Source: three-view drawing plus pictorial views. Frame: mm from the lowest corner of the part. A direction names the side the tool comes from. Give positions to 0.01 mm unless a question says otherwise; leave off trailing zeros. Loops run counter-clockwise (first coordinate to the right, second up) from the corner with the lowest first, then second, coordinate; pieces in that order, holes last. Notation, with made-up numbers: (-17, 82) -> (-10, 82) arc R23 cw to (-10, 101) -> close; hole circle Ø6 at (44.25, -11.5). An arc over 180 degrees is marked (long way). One line per item, written item: value. Start each with the question number.
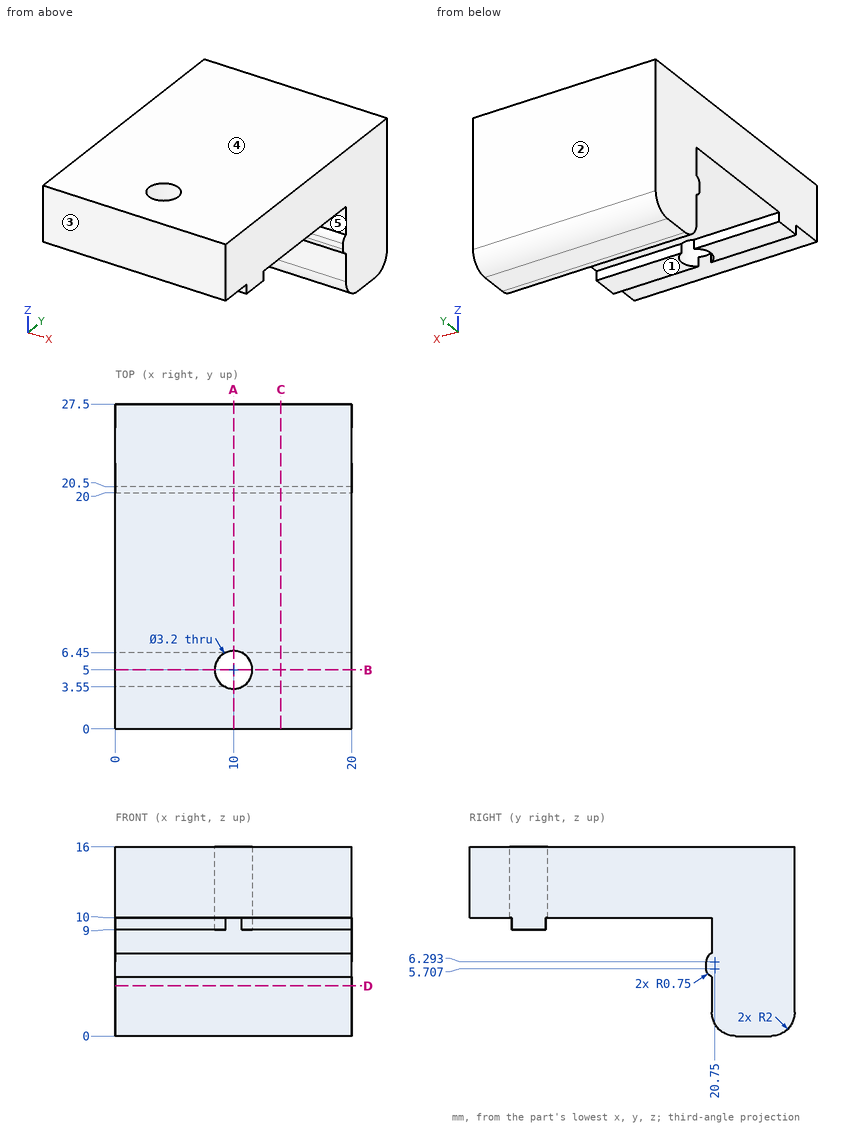
Item 1: Access query for the marked faces 1 and 2. Directions: +Z, -Z, +X, -X, +Y, -Y. A direction counts if a zero-diameter tool reaches every point of the face in a straight line with its end or side. Return the directions, or none.
Item 2: Pin query (flat end, axial travel): pin 1 (5 mm diameter, centred on x = 10, y = 5, fed in from -Z); pin 2 (0.5 mm diameter, centred on x = 5, z = 9.5, fed in from -Y); pin 3 (0.5 mm diameter, centred on x = 13.5, z = 6, fed in from -Y). Return the tip coordinate at first contact, or that it passes through.
Item 3: Section C-C, the plane x = 14. Output: boundary loops of the cut face in (y, z), then the cut area to 3 significant figures.
Item 4: Mould query, pull axis Y, two halves, no side actions, for the marked faces 3, 4 and 5. Classes: pulls with the +Y half, pulls with the -Y half, needs draft (parallel to the pull), parting line crosses it, or undercut.
Item 5: Section D-D, the plane z = 4.25. Output: boundary loops of the cut face in (x, y).
Item 6: Section A-A, the plane x = 10. Output: boundary loops of the cut face in (y, z), then the cut area to 3 significant figures.
Item 7: Ray query, line 1 along Y through (x, z) = (10, 13); line 2 along Y through (x, z) = (2.5, 9.75); line 3 along Y through (x, z) = (10.25, 2). Return the intervals inside material, ascending. Write a range as [from, to].
Item 8: Section B-B, the plane y = 5. Output: boundary loops of the cut face in (x, z), then the cut area to 3 significant figures.
Geometry check:
1. face 1: -Z, +X, -X, -Y
1. face 2: +Z, -Z, +X, -X, +Y
2. pin 1: stops at z = 9
2. pin 2: stops at y = 3.55
2. pin 3: stops at y = 20
3. outline: (0, 10) -> (3.55, 10) -> (3.55, 9) -> (6.45, 9) -> (6.45, 10) -> (20.5, 10) -> (20.5, 7) arc R0.75 ccw to (20, 6.29) -> (20, 5.71) arc R0.75 ccw to (20.5, 5) -> (20.5, 2) arc R2 ccw to (22.5, 0) -> (25.5, 0) arc R2 ccw to (27.5, 2) -> (27.5, 16) -> (0, 16) -> close
3. area: 237 mm2
4. face 3: pulls with the -Y half
4. face 4: needs draft
4. face 5: undercut
5. outline: (0, 20.5) -> (20, 20.5) -> (20, 27.5) -> (0, 27.5) -> close
6. outline: (0, 10) -> (3.4, 10) -> (3.4, 16) -> (0, 16) -> close; (6.6, 10) -> (20.5, 10) -> (20.5, 7) arc R0.75 ccw to (20, 6.29) -> (20, 5.71) arc R0.75 ccw to (20.5, 5) -> (20.5, 2) arc R2 ccw to (22.5, 0) -> (25.5, 0) arc R2 ccw to (27.5, 2) -> (27.5, 16) -> (6.6, 16) -> close
6. area: 215 mm2
7. line 1: y = [0, 3.4], [6.6, 27.5]
7. line 2: y = [3.55, 6.45], [20.5, 27.5]
7. line 3: y = [20.5, 27.5]
8. outline: (0, 9) -> (8.4, 9) -> (8.4, 16) -> (0, 16) -> close; (11.6, 9) -> (20, 9) -> (20, 16) -> (11.6, 16) -> close
8. area: 118 mm2
